Here's the drawing with two shaded views (mm, measured from the low corner). I have some questions. Give positions to 0.01 mm unless a question says otherwise; leave off trailing zeros. Loops run counter-clockwise (first coordinate to the right, second up) from the corner with the lowest first, then second, coordinate; pieces in that order, holes last.
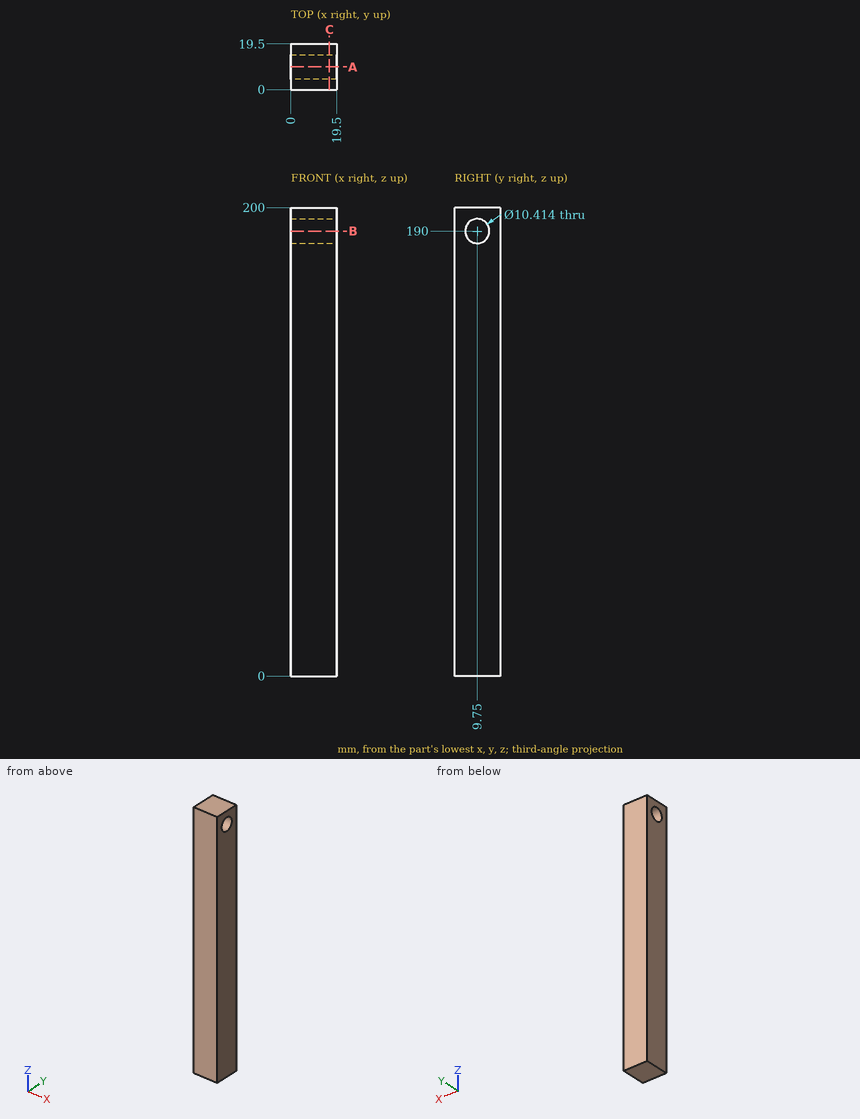
(1) Please list where these lines run through material, in increasing order: probe 1 along Y at (x, z) = (11.25, 190); probe 2 along Z at (x, y) = (13.25, 9.75); probe 3 along Z at (x, y) = (14.75, 14.5) (1 decimal).
Returned:
probe 1: y = 0 to 4.54, 14.96 to 19.5
probe 2: z = 0 to 184.79, 195.21 to 200
probe 3: z = 0 to 187.9, 192.1 to 200
(2) Suppose I cut it at B-B on z = 190. List the corners of the cut face in (x, y) for me, plus the area to 3 significant figures.
Returned:
outline: (0, 0) - (19.5, 0) - (19.5, 4.54) - (0, 4.54) - close; (0, 14.96) - (19.5, 14.96) - (19.5, 19.5) - (0, 19.5) - close
area: 177 mm2
(3) Suppose I cut it at C-C on x = 16.5. List the corners of the cut face in (y, z) for me.
Returned:
outline: (0, 0) - (19.5, 0) - (19.5, 200) - (0, 200) - close; hole circle Ø10.41 at (9.75, 190)
(4) Suppose I cut it at A-A on y = 9.75. List the corners of the cut face in (x, z) for me, plus the area to 3 significant figures.
Returned:
outline: (0, 0) - (19.5, 0) - (19.5, 184.79) - (0, 184.79) - close; (0, 195.21) - (19.5, 195.21) - (19.5, 200) - (0, 200) - close
area: 3,700 mm2
